Geometry check sheet. Reference: the model listing, model coordinates, mm. Face numbers are marked on the shaded views. A direction names the side the tool comes from. Coordinates: 2 decimals unless noted, no trailing zeros. Order: outer loops, then holes, each group sorted by start corner. A loop starts at its lowest first (then second) coordinate and runs counter-clockwise, first axis right, second up. Notation, with made-up numbers: (-6, 68) -> (21, 68) arc R16 ccw to (21, 74) -> close; hole circle Ø3 at (3, 65.5). An arc over 180 degrees is marked (long way). Answer in a Markdown table with one row per item. Add a question column.
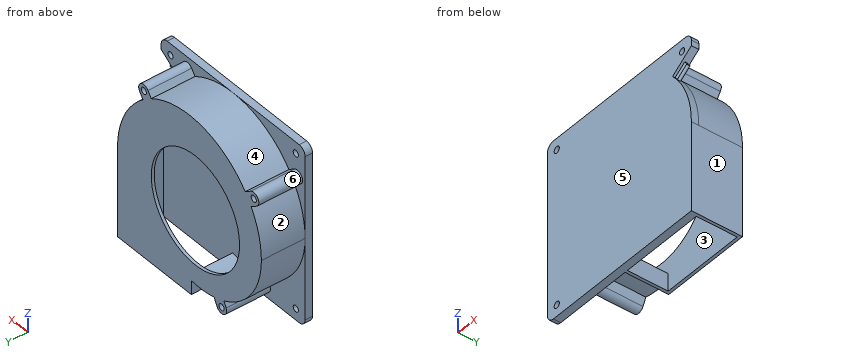
```python
from build123d import *

# Parameters (mm, degrees)
ESBO_O1_W                = 120.6
ESBO_O1_H                = 120.6
RESSALTO_EXTRUS_O1_DEPTH = 5
ESBO_O2_R                = 2.16
ESBO_O2_R_2              = 37
RESSALTO_EXTRUS_O2_DEPTH = 29.48
CORTE_EXTRUS_O1_DEPTH    = 27.48
CORTE_EXTRUS_O2_REACH    = 92.229
ESBO_O4_R                = 2.175
CORTE_EXTRUS_O3_REACH    = 92.229
FILETE1_R                = 5
ESBO_O6_R                = 1
RESSALTO_EXTRUS_O3_DEPTH = 10


with BuildPart() as part:
    # Esboço1 → Ressalto-extrusão1 (new body)
    with BuildSketch(Plane(origin=(0, 0, 0), x_dir=(1, 0, 0), z_dir=(0, 1, 0))):
        Rectangle(ESBO_O1_W, ESBO_O1_H)
    extrude(amount=RESSALTO_EXTRUS_O1_DEPTH)

    # Esboço2 → Ressalto-extrusão2 (add)
    with BuildSketch(Plane(origin=(0, 5, 0), x_dir=(1, 0, 0), z_dir=(0, 1, 0))):
        with BuildLine():
            Line((-1.55, 60.3), (-1.55, 50.74))
            ThreePointArc((-1.55, 50.74), (-11.149709748, 51.241553514), (-20.674386419, 49.942893633))
            Line((-20.674386419, 49.942893633), (-23.114662996, 54.72290087))
            ThreePointArc((-23.114662996, 54.72290087), (-28.89290087, 56.595337004), (-30.765337004, 50.81709913))
            Line((-30.765337004, 50.81709913), (-28.946397101, 47.25416451))
            ThreePointArc((-28.946397101, 47.25416451), (-51.748686365, 28.3549135), (-60.3, 0))
            ThreePointArc((-60.3, 0), (-58.11119265, -16.099046207), (-51.703672015, -31.029345791))
            Line((-51.703672015, -31.029345791), (-56.356828802, -34.294067597))
            ThreePointArc((-56.356828802, -34.294067597), (-57.405932403, -40.276828802), (-51.423171198, -41.325932403))
            Line((-51.423171198, -41.325932403), (-46.77001441, -38.061210596))
            ThreePointArc((-46.77001441, -38.061210596), (-9.861567273, -59.488145802), (31.986619032, -51.116985464))
            Line((31.986619032, -51.116985464), (34.770606047, -54.931863068))
            ThreePointArc((34.770606047, -54.931863068), (40.771863068, -55.869393953), (41.709393953, -49.868136932))
            Line((41.709393953, -49.868136932), (38.925406938, -46.053259327))
            ThreePointArc((38.925406938, -46.053259327), (54.695941524, -25.385901221), (60.3, 0))
            Line((60.3, 0), (60.3, 60.3))
            Line((60.3, 60.3), (-1.55, 60.3))
        make_face()
        with Locations(Location((-53.89, -37.81, 0), (0, 0, 270))):
            Circle(ESBO_O2_R, mode=Mode.SUBTRACT)
        with Locations(Location((38.24, -52.4, 0), (0, 0, 270))):
            Circle(ESBO_O2_R, mode=Mode.SUBTRACT)
        with Locations(Location((-5.011670261, 1.136043404, 0), (0, 0, 270))):
            Circle(ESBO_O2_R_2, mode=Mode.SUBTRACT)
        with Locations(Location((-26.94, 52.77, 0), (0, 0, 270))):
            Circle(ESBO_O2_R, mode=Mode.SUBTRACT)
    extrude(amount=RESSALTO_EXTRUS_O2_DEPTH)

    # Esboço3 → Corte-extrusão1 (cut)
    with BuildSketch(Plane(origin=(0, 5, 0), x_dir=(1, 0, 0), z_dir=(0, 1, 0))):
        with BuildLine():
            Line((58.3, 60.3), (0.45, 60.3))
            Line((0.45, 60.3), (0.45, 48.368870154))
            ThreePointArc((0.45, 48.368870154), (-10.684091117, 49.257737718), (-21.732404969, 47.616752781))
            ThreePointArc((-21.732404969, 47.616752781), (-48.103316228, 30.018927995), (-58.3, 0))
            ThreePointArc((-58.3, 0), (-55.237005698, -18.64841016), (-46.369873019, -35.337301485))
            ThreePointArc((-46.369873019, -35.337301485), (-7.26299238, -57.845820434), (36.194519906, -45.703902774))
            ThreePointArc((36.194519906, -45.703902774), (52.483476021, -25.384537513), (58.3, 0))
            Line((58.3, 0), (58.3, 60.3))
        make_face()
    extrude(amount=CORTE_EXTRUS_O1_DEPTH, mode=Mode.SUBTRACT)

    # Esboço4 → Corte-extrusão2 (cut, up to next)
    with BuildSketch(Plane(origin=(0, 5, 0), x_dir=(1, 0, 0), z_dir=(0, 1, 0)), mode=Mode.PRIVATE) as corte_extrus_o2_sk1:
        with Locations(Location((-52.525, 52.525, 0), (0, 0, 270))):
            Circle(ESBO_O4_R)
    corte_extrus_o2_tool1 = extrude(corte_extrus_o2_sk1.sketch, amount=-CORTE_EXTRUS_O2_REACH, mode=Mode.PRIVATE) & part.part
    # Esboço4 → Corte-extrusão2 (cut, up to next)
    with BuildSketch(Plane(origin=(0, 5, 0), x_dir=(1, 0, 0), z_dir=(0, 1, 0)), mode=Mode.PRIVATE) as corte_extrus_o2_sk2:
        with Locations(Location((-52.525, -52.525, 0), (0, 0, 270))):
            Circle(ESBO_O4_R)
    corte_extrus_o2_tool2 = extrude(corte_extrus_o2_sk2.sketch, amount=-CORTE_EXTRUS_O2_REACH, mode=Mode.PRIVATE) & part.part
    # Esboço4 → Corte-extrusão2 (cut, up to next)
    with BuildSketch(Plane(origin=(0, 5, 0), x_dir=(1, 0, 0), z_dir=(0, 1, 0)), mode=Mode.PRIVATE) as corte_extrus_o2_sk3:
        with Locations(Location((52.525, -52.525, 0), (0, 0, 270))):
            Circle(ESBO_O4_R)
    corte_extrus_o2_tool3 = extrude(corte_extrus_o2_sk3.sketch, amount=-CORTE_EXTRUS_O2_REACH, mode=Mode.PRIVATE) & part.part
    add(corte_extrus_o2_tool1.solids().sort_by_distance((-52.525, 5, -52.525))[0], mode=Mode.SUBTRACT)
    add(corte_extrus_o2_tool2.solids().sort_by_distance((-52.525, 5, 52.525))[0], mode=Mode.SUBTRACT)
    add(corte_extrus_o2_tool3.solids().sort_by_distance((52.525, 5, 52.525))[0], mode=Mode.SUBTRACT)

    # Esboço5 → Corte-extrusão3 (cut, up to next)
    with BuildSketch(Plane(origin=(0, 5, 0), x_dir=(1, 0, 0), z_dir=(0, 1, 0)), mode=Mode.PRIVATE) as corte_extrus_o3_sk1:
        with BuildLine():
            Line((44.583965728, -40.6), (60.3, -51.5))
            Line((60.3, -51.5), (60.3, 0))
            ThreePointArc((60.3, 0), (56.233900511, -21.767830239), (44.583965728, -40.6))
        make_face()
    corte_extrus_o3_tool1 = extrude(corte_extrus_o3_sk1.sketch, amount=-CORTE_EXTRUS_O3_REACH, mode=Mode.PRIVATE) & part.part
    add(corte_extrus_o3_tool1.solids().sort_by_distance((55.517815, 5, 34.778599))[0], mode=Mode.SUBTRACT)

    # Filete1
    filete1_edges = [part.edges().sort_by_distance(p)[0] for p in [
        (-60.3, 2.5, -60.3),
        (60.3, 2.5, 60.3),
        (-60.3, 2.5, 60.3),
    ]]
    fillet(filete1_edges, radius=FILETE1_R)

    # Esboço6 → Ressalto-extrusão3 (add)
    with BuildSketch(Plane(origin=(49.116321983, 0, 34.065076491), x_dir=(0, 1, 0), z_dir=(-0.8217106210842787, 1.9312545644066756e-15, -0.5699049527748369))):
        with Locations(Location((1.975912972, -6.452828334, 0), (0, 0, 270))):
            Circle(ESBO_O6_R)
        with Locations(Location((1.975912972, -3.452828334, 0), (0, 0, 270))):
            Circle(ESBO_O6_R)
    extrude(amount=-RESSALTO_EXTRUS_O3_DEPTH)


solid = part.part
```
(1) Cross-section at D-D (x = -9). Enter the section's corners in (y, z), plus the area to 3 significant figures.
(2) Cross-section at A-A (y = 11). Enter the section's corners in (x, z) (3 decimals), plus the area to 3 significant figures.
(3) Mould release check, pull along Z, two halves, no side actions. Record for the marked faces 4, 5 and 6: +Z half, -Z half, draft (parallel to the pull), parting line (faces both ways), or undercut.
(4) Cross-section at B-B (z = -52.77). Enter the section's corners in (x, y) (3 decimals), plus the area to 3 significant figures.
(5) Go/stop test with flat-tipped pins: P1, Ø5, axis at y = 17.5, z = 7, coming from the +X side; P2, Ø1.5, axis at x = 14.5, y = 23.5, coming from the +Z side; P3, Ø3, axis at x = -39, y = 21.5, coming from the -Z side; P4, Ø3.5, axis at x = -52.525, z = -52.525, coming from the +Y side. Record where each tip stops, or that it passes through.
(6) Scan lines: line 1 along Y through (x, z) = (39, -40); line 2 along Z through (x, y) = (-53, 22); line 3 along Y through (x, z) = (7, 24.5). Record each from-to range of solid material in increasing order.
(7) Cross-section at C-C (x = 8). Enter the section's corners in (y, z), plus the area to 3 significant figures.
(8) Access from +Z, -Z, +X, -X, +Y, -Y to the whole of each face (thin tool, end or side, straight path). Record for the marked faces 1, 2 and 3.
Checks:
| question | item | result |
|---|---|---|
| 1 | outline | (0, -60.3) -> (5, -60.3) -> (5, -51.29) -> (34.48, -51.29) -> (34.48, -37.92) -> (32.48, -37.92) -> (32.48, -49.29) -> (5, -49.29) -> (5, 57.6) -> (32.48, 57.6) -> (32.48, 35.65) -> (34.48, 35.65) -> (34.48, 59.62) -> (5, 59.62) -> (5, 60.3) -> (0, 60.3) -> close |
| 1 | area | 788 mm² |
| 2 | outline | (-60.3, 0) arc R51.286 ccw to (-28.946, -47.254) -> (-30.765, -50.817) arc R4.295 ccw to (-23.115, -54.723) -> (-20.674, -49.943) arc R51.286 ccw to (-1.55, -50.74) -> (-1.55, -60.3) -> (0.45, -60.3) -> (0.45, -48.369) arc R49.286 cw to (-58.3, 0) arc R58.3 cw to (58.3, 0) -> (58.3, -60.3) -> (60.3, -60.3) -> (60.3, 0) arc R60.3 ccw to (38.925, 46.053) -> (41.709, 49.868) arc R4.295 ccw to (34.771, 54.932) -> (31.987, 51.117) arc R60.3 ccw to (-46.77, 38.061) -> (-51.423, 41.326) arc R4.295 ccw to (-56.357, 34.294) -> (-51.704, 31.029) arc R60.3 ccw to start; hole circle Ø4.32 at (-53.89, 37.81); hole circle Ø4.32 at (-26.94, -52.77); hole circle Ø4.32 at (38.24, 52.4) |
| 2 | area | 859 mm² |
| 3 | face 4 | +Z half |
| 3 | face 5 | draft |
| 3 | face 6 | undercut |
| 4 | outline | (-60.3, 0) -> (-54.686, 0) -> (-54.686, 5) -> (-60.3, 5) -> close; (-50.364, 0) -> (60.3, 0) -> (60.3, 34.48) -> (-1.55, 34.48) -> (-1.55, 5) -> (-22.118, 5) -> (-22.118, 34.48) -> (-24.78, 34.48) -> (-24.78, 5) -> (-29.1, 5) -> (-29.1, 34.48) -> (-31.235, 34.48) -> (-31.235, 5) -> (-50.364, 5) -> close; hole (0.45, 5) -> (58.3, 5) -> (58.3, 32.48) -> (0.45, 32.48) -> close |
| 4 | area | 956 mm² |
| 5 | P1 | x = 60.13 |
| 5 | P2 | z = 58.71 |
| 5 | P3 | z = -42.65 |
| 5 | P4 | through |
| 6 | line 1 | 0 to 5, 32.48 to 34.48 |
| 6 | line 2 | -26.37 to -22.23, 24.29 to 28.76, 31.94 to 35.84, 39.78 to 42.01 |
| 6 | line 3 | 0 to 5 |
| 7 | outline | (0, -60.3) -> (5, -60.3) -> (5, 57.75) -> (32.48, 57.75) -> (32.48, 33.5) -> (34.48, 33.5) -> (34.48, 59.77) -> (5, 59.77) -> (5, 60.3) -> (0, 60.3) -> close; (32.48, -60.3) -> (34.48, -60.3) -> (34.48, -35.77) -> (32.48, -35.77) -> close |
| 7 | area | 760 mm² |
| 8 | face 1 | +Z, -Z, +X, +Y, -Y |
| 8 | face 2 | -X, +Y |
| 8 | face 3 | none |
